Could you check a few things on this model? Use its own coordinates, in mm. Face numbers are marked on the shaded views. A direction names the side the tool comes from. Round coordinates to 2 decimals unless told otherwise and drop trailing zeros. Loops run counter-clockwise (first coordinate to the right, second up) from the corner with the lowest first, then second, coordinate; pieces in that order, holes last. Notation, with made-up numbers: M 79.5,13 L 130.5,13 A33 cw 130.5,46 Z; hole C -29,-4.75 d10. An arc over 180 degrees is marked long. Return JSON: item names as keys, results as strings. Group by question number.
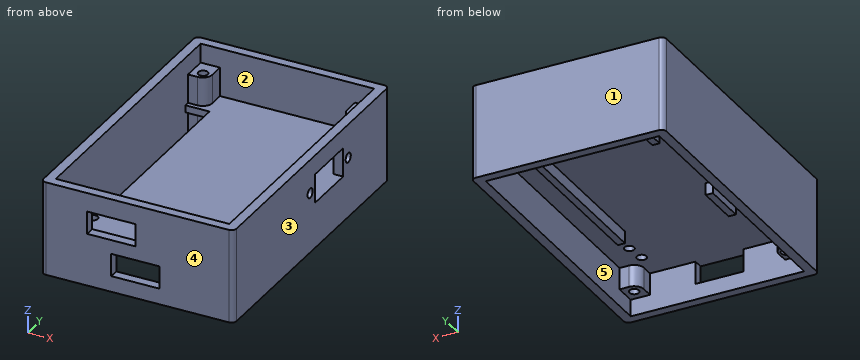
```python
from build123d import *

# Parameters (mm, degrees)
SKETCH_2_R             = 1
EXTRUDE_2250_DEPTH     = 7.5
EXTRUDE_2250_2_DEPTH   = 7.5
EXTRUDE_2250_3_DEPTH   = 7.5
EXTRUDE_2250_4_DEPTH   = 7.5
EXTRUDE_START          = -4.5
SKETCH_2_5_R           = 1
EXTRUDE_2650_DEPTH     = 4.5
EXTRUDE_2650_2_DEPTH   = 4.5
EXTRUDE_2650_3_DEPTH   = 4.5
EXTRUDE_2650_4_DEPTH   = 4.5
EXTRUDE_2769_DEPTH     = 11.5
SKETCH_15_W            = 10
SKETCH_15_H            = 4.7
CUT_EXTRUDE_2936_DEPTH = 2
ESP32_START            = -8
ESP32_DEPTH            = 8
ESP32_3_W              = 10
ESP32_3_H              = 4.7
ESP32_2_DEPTH          = 2
SKETCH_1_29_R          = 1
SKETCH_1_29_W          = 1.5
SKETCH_1_29_H          = 9
EXTRUDE_3195_DEPTH     = 1.5
EXTRUDE_3_DEPTH        = 2.5
SKETCH_1_30_W          = 1.5
SKETCH_1_30_H          = 9
EXTRUDE_3_2_DEPTH      = 2.5
SKETCH_1_31_W          = 1.5
SKETCH_1_31_H          = 9
EXTRUDE_4_DEPTH        = 1.5
SKETCH_18_R            = 1
SKETCH_18_W            = 6
SKETCH_18_H            = 11
CUT_EXTRUDE_4645_DEPTH = 2


with BuildPart() as part:
    # Sketch 2 → Extrude 2250 (new body)
    with BuildSketch(Plane.XY):
        with BuildLine():
            Line((0, 0), (4, 0))
            Line((4, 0), (4, 2.4))
            ThreePointArc((4, 2.4), (3.414213562, 3.814213562), (2, 4.4))
            Line((2, 4.4), (0, 4.4))
            Line((0, 4.4), (0, 0))
        make_face()
        with Locations((2.5, 2.4)):
            Circle(SKETCH_2_R, mode=Mode.SUBTRACT)
    extrude(amount=EXTRUDE_2250_DEPTH)



with BuildPart() as body_2:
    # Sketch 2 → Extrude 2250 2 (new body)
    with BuildSketch(Plane.XY):
        with BuildLine():
            Line((36, 0), (32, 0))
            Line((32, 0), (32, 2.4))
            ThreePointArc((32, 2.4), (32.585786438, 3.814213562), (34, 4.4))
            Line((34, 4.4), (36, 4.4))
            Line((36, 4.4), (36, 0))
        make_face()
        with Locations((34, 2.4)):
            Circle(SKETCH_2_R, mode=Mode.SUBTRACT)
    extrude(amount=EXTRUDE_2250_2_DEPTH)


with BuildPart() as body_3:
    # Sketch 2 → Extrude 2250 3 (new body)
    with BuildSketch(Plane.XY):
        with BuildLine():
            Line((36, 57), (32, 57))
            Line((32, 57), (32, 54))
            ThreePointArc((32, 54), (32.585786438, 52.585786438), (34, 52))
            Line((34, 52), (36, 52))
            Line((36, 52), (36, 57))
        make_face()
        with Locations((33.75, 53.699390835)):
            Circle(SKETCH_2_R, mode=Mode.SUBTRACT)
    extrude(amount=EXTRUDE_2250_3_DEPTH)


with BuildPart() as body_4:
    # Sketch 2 → Extrude 2250 4 (new body)
    with BuildSketch(Plane.XY):
        with BuildLine():
            Line((0, 57), (4, 57))
            Line((4, 57), (4, 54))
            ThreePointArc((4, 54), (3.414213562, 52.585786438), (2, 52))
            Line((2, 52), (0, 52))
            Line((0, 52), (0, 57))
        make_face()
        with Locations((2.25, 53.699390835)):
            Circle(SKETCH_2_R, mode=Mode.SUBTRACT)
    extrude(amount=EXTRUDE_2250_4_DEPTH)


with BuildPart() as body_5:
    # Sketch 2_5 → Extrude 2650 (new body)
    with BuildSketch(Plane.XY.offset(EXTRUDE_START)):
        with BuildLine():
            Line((0, 0), (4, 0))
            Line((4, 0), (4, 2.4))
            ThreePointArc((4, 2.4), (3.414213562, 3.814213562), (2, 4.4))
            Line((2, 4.4), (0, 4.4))
            Line((0, 4.4), (0, 0))
        make_face()
        with Locations((2.5, 2.4)):
            Circle(SKETCH_2_5_R, mode=Mode.SUBTRACT)
    extrude(amount=EXTRUDE_2650_DEPTH)


with BuildPart() as body_6:
    # Sketch 2_5 → Extrude 2650 2 (new body)
    with BuildSketch(Plane.XY.offset(EXTRUDE_START)):
        with BuildLine():
            Line((36, 0), (32, 0))
            Line((32, 0), (32, 2.4))
            ThreePointArc((32, 2.4), (32.585786438, 3.814213562), (34, 4.4))
            Line((34, 4.4), (36, 4.4))
            Line((36, 4.4), (36, 0))
        make_face()
        with Locations((34, 2.4)):
            Circle(SKETCH_2_5_R, mode=Mode.SUBTRACT)
    extrude(amount=EXTRUDE_2650_2_DEPTH)


with BuildPart() as body_7:
    # Sketch 2_5 → Extrude 2650 3 (new body)
    with BuildSketch(Plane.XY.offset(EXTRUDE_START)):
        with BuildLine():
            Line((36, 57), (32, 57))
            Line((32, 57), (32, 54))
            ThreePointArc((32, 54), (32.585786438, 52.585786438), (34, 52))
            Line((34, 52), (36, 52))
            Line((36, 52), (36, 57))
        make_face()
        with Locations((33.75, 53.699390835)):
            Circle(SKETCH_2_5_R, mode=Mode.SUBTRACT)
    extrude(amount=EXTRUDE_2650_3_DEPTH)


with BuildPart() as body_8:
    # Sketch 2_5 → Extrude 2650 4 (new body)
    with BuildSketch(Plane.XY.offset(EXTRUDE_START)):
        with BuildLine():
            Line((0, 57), (4, 57))
            Line((4, 57), (4, 54))
            ThreePointArc((4, 54), (3.414213562, 52.585786438), (2, 52))
            Line((2, 52), (0, 52))
            Line((0, 52), (0, 57))
        make_face()
        with Locations((2.25, 53.699390835)):
            Circle(SKETCH_2_5_R, mode=Mode.SUBTRACT)
    extrude(amount=EXTRUDE_2650_4_DEPTH)


with BuildPart() as part_1:
    add(part.part)

    add(body_2.part)  # Extrude 2769 merges body 2

    add(body_3.part)  # Extrude 2769 merges body 3

    add(body_4.part)  # Extrude 2769 merges body 4

    add(body_5.part)  # Extrude 2769 merges body 5

    add(body_6.part)  # Extrude 2769 merges body 6

    add(body_7.part)  # Extrude 2769 merges body 7

    add(body_8.part)  # Extrude 2769 merges body 8
    # Sketch 1 → Extrude 2769 (add)
    with BuildSketch(Plane.XY):
        with BuildLine():
            ThreePointArc((-2, -1), (-1.707106781, -1.707106781), (-1, -2))
            Line((-1, -2), (37, -2))
            ThreePointArc((37, -2), (37.707106781, -1.707106781), (38, -1))
            Line((38, -1), (38, 58))
            ThreePointArc((38, 58), (37.707106781, 58.707106781), (37, 59))
            Line((37, 59), (-1, 59))
            ThreePointArc((-1, 59), (-1.707106781, 58.707106781), (-2, 58))
            Line((-2, 58), (-2, -1))
        make_face()
        Polygon((36, 0), (0, 0), (0, 15), (0, 51), (0, 57), (36, 57), align=None, mode=Mode.SUBTRACT)
    extrude(amount=EXTRUDE_2769_DEPTH)

    # Sketch 15 → Cut-Extrude 2936 (cut)
    with BuildSketch(Plane.XZ):
        with Locations((12.56, 5.25)):
            Rectangle(SKETCH_15_W, SKETCH_15_H)
    extrude(amount=CUT_EXTRUDE_2936_DEPTH, mode=Mode.SUBTRACT)

    # Sketch 1 regions → ESP32 (add)
    with BuildSketch(Plane.XY.offset(ESP32_START)):
        with BuildLine():
            ThreePointArc((-2, -1), (-1.707106781, -1.707106781), (-1, -2))
            Line((-1, -2), (37, -2))
            ThreePointArc((37, -2), (37.707106781, -1.707106781), (38, -1))
            Line((38, -1), (38, 58))
            ThreePointArc((38, 58), (37.707106781, 58.707106781), (37, 59))
            Line((37, 59), (-1, 59))
            ThreePointArc((-1, 59), (-1.707106781, 58.707106781), (-2, 58))
            Line((-2, 58), (-2, -1))
        make_face()
        Polygon((36, 0), (0, 0), (0, 15), (0, 51), (0, 57), (36, 57), align=None, mode=Mode.SUBTRACT)
    extrude(amount=ESP32_DEPTH)

    # ESP32 3 → ESP32 2 (cut)
    with BuildSketch(Plane(origin=(0, 0, 0), x_dir=(1, 0, 0), z_dir=(0, 1, 0))):
        with Locations((17.56, 2.35)):
            Rectangle(ESP32_3_W, ESP32_3_H)
    extrude(amount=-ESP32_2_DEPTH, mode=Mode.SUBTRACT)

    # Sketch 1_29 → Extrude 3195 (add)
    with BuildSketch(Plane.XY):
        Polygon((0, 15), (0, 0), (36, 0), (36, 57), (0, 57), (0, 51), (5, 51), (5, 15), align=None)
        with Locations((4.56, 6)):
            Circle(SKETCH_1_29_R, mode=Mode.SUBTRACT)
        with Locations((4, 10)):
            Circle(SKETCH_1_29_R, mode=Mode.SUBTRACT)
        with Locations((6.5, 20.5)):
            Rectangle(SKETCH_1_29_W, SKETCH_1_29_H, mode=Mode.SUBTRACT)
        with Locations((30.56, 6)):
            Circle(SKETCH_1_29_R, mode=Mode.SUBTRACT)
        with Locations((31, 10)):
            Circle(SKETCH_1_29_R, mode=Mode.SUBTRACT)
        Polygon((30.25, 16), (28.75, 16), (28.75, 52), (7.25, 52), (7.25, 46), (5.75, 46), (5.75, 53.5), (30.25, 53.5), (30.25, 52), align=None, mode=Mode.SUBTRACT)
    extrude(amount=EXTRUDE_3195_DEPTH)



with BuildPart() as body_2_2:
    # Sketch 1_30 → Extrude 3 (new body)
    with BuildSketch(Plane.XY):
        Polygon((5.75, 46), (7.25, 46), (7.25, 52), (28.75, 52), (28.75, 16), (30.25, 16), (30.25, 52), (30.25, 53.5), (5.75, 53.5), align=None)
    extrude(amount=-EXTRUDE_3_DEPTH)


with BuildPart() as body_3_2:
    # Sketch 1_30 → Extrude 3 2 (new body)
    with BuildSketch(Plane.XY):
        with Locations((6.5, 20.5)):
            Rectangle(SKETCH_1_30_W, SKETCH_1_30_H)
    extrude(amount=-EXTRUDE_3_2_DEPTH)


with BuildPart() as part_2:
    add(part_1.part)

    add(body_2_2.part)  # Extrude 4 merges body 2 2

    add(body_3_2.part)  # Extrude 4 merges body 3 2
    # Sketch 1_31 → Extrude 4 (add)
    with BuildSketch(Plane.XY):
        Polygon((28.75, 16), (30.25, 16), (30.25, 52), (30.25, 53.5), (5.75, 53.5), (5.75, 46), (7.25, 46), (7.25, 52), (28.75, 52), align=None)
        with Locations((6.5, 20.5)):
            Rectangle(SKETCH_1_31_W, SKETCH_1_31_H)
    extrude(amount=EXTRUDE_4_DEPTH)

    # Sketch 18 → Cut-Extrude 4645 (cut)
    with BuildSketch(Plane(origin=(38, 0, 0), x_dir=(0, 0, -1), z_dir=(1, 0, 0))):
        with Locations((-4.5, 43)):
            Circle(SKETCH_18_R)
        with Locations((-4.5, 28)):
            Circle(SKETCH_18_R)
        with Locations((-4.5, 35.5)):
            Rectangle(SKETCH_18_W, SKETCH_18_H)
    extrude(amount=-CUT_EXTRUDE_4645_DEPTH, mode=Mode.SUBTRACT)


solid = part_2.part
```
1. We'd pull the mould along Y, two halves only. Please class the marked faces 1, 2 and 3: +Y half, -Y half, draft (parallel to the pull), parting line (faces both ways), or undercut.
2. If we section it at C-C, the plane x = 19: Please give me the cut outline in (y, z), then the cut area to 3 significant figures.
3. If we section it at A-A, the plane z = 10: Please give me the cut outline in (x, y).
4. I need wall thicknesses on probe 1 along Y at (x, z) = (5.5, 9.75); probe 2 along X at (y, z) = (13, 8.75); probe 3 along Y at (x, z) = (4, 0.6). Which ranges of each line are inside material? Lowest first, please.
5. I'm going to push flat-ended pins straight in: pin 1 Ø2 at (x, y) = (2.5, 3) entering from +Z; pin 2 Ø1.5 at (x, y) = (11.5, 23.5) entering from +Z; pin 3 Ø1.6 at (x, y) = (33.75, 53.7) entering from -Z. Where does each tip first touch, or does it pass through?
6. On a 3-axis mill with a long thin cutter (end or side, diameter ignored), from which of +Z, -Z, +X, -X, +Y, -Y can I reach the whole of each face in a straight line? I mean the marked faces 4 and 5. Say none if no direction works.
7. If we section it at D-D, the plane x = 13.5: Please give me the cut outline in (y, z), then the cut area to 3 significant figures.
8. If we section it at B-B, the plane y = 6: Please give me the cut outline in (x, z).
Geometry results:
{
 "1": {"face 1": "+Y half", "face 2": "undercut", "face 3": "draft"},
 "2": {"outline": "M -2,-8 L 0,-8 L 0,-4.7 L -2,-4.7 Z; M -2,0 L 52,0 L 52,-2.5 L 53.5,-2.5 L 53.5,0 L 57,0 L 57,-8 L 59,-8 L 59,11.5 L 57,11.5 L 57,1.5 L 0,1.5 L 0,11.5 L -2,11.5 Z", "area": "158 mm^2"},
 "3": {"outline": "M -2,-1 A1 ccw -1,-2 L 37,-2 A1 ccw 38,-1 L 38,58 A1 ccw 37,59 L -1,59 A1 ccw -2,58 Z; hole M 0,0 L 36,0 L 36,57 L 0,57 Z"},
 "4": {"probe 1": "-2 to 0, 57 to 59", "probe 2": "-2 to 0, 36 to 38", "probe 3": "-2 to 5.17, 6.83 to 9, 11 to 15, 51 to 59"},
 "5": {"pin 1": "z = 7.5", "pin 2": "z = 1.5", "pin 3": "z = 0"},
 "6": {"face 4": "+Z, -Z, +X, -X, -Y", "face 5": "-Z"},
 "7": {"outline": "M -2,-8 L 0,-8 L 0,-4.7 L -2,-4.7 Z; M -2,0 L 52,0 L 52,-2.5 L 53.5,-2.5 L 53.5,0 L 57,0 L 57,-8 L 59,-8 L 59,11.5 L 57,11.5 L 57,1.5 L 0,1.5 L 0,2.9 L -2,2.9 Z; M -2,7.6 L 0,7.6 L 0,11.5 L -2,11.5 Z", "area": "148 mm^2"},
 "8": {"outline": "M -2,-8 L 0,-8 L 0,0 L 3.56,0 L 3.56,1.5 L 0,1.5 L 0,11.5 L -2,11.5 Z; M 5.56,0 L 29.56,0 L 29.56,1.5 L 5.56,1.5 Z; M 31.56,0 L 36,0 L 36,-8 L 38,-8 L 38,11.5 L 36,11.5 L 36,1.5 L 31.56,1.5 Z"}
}
